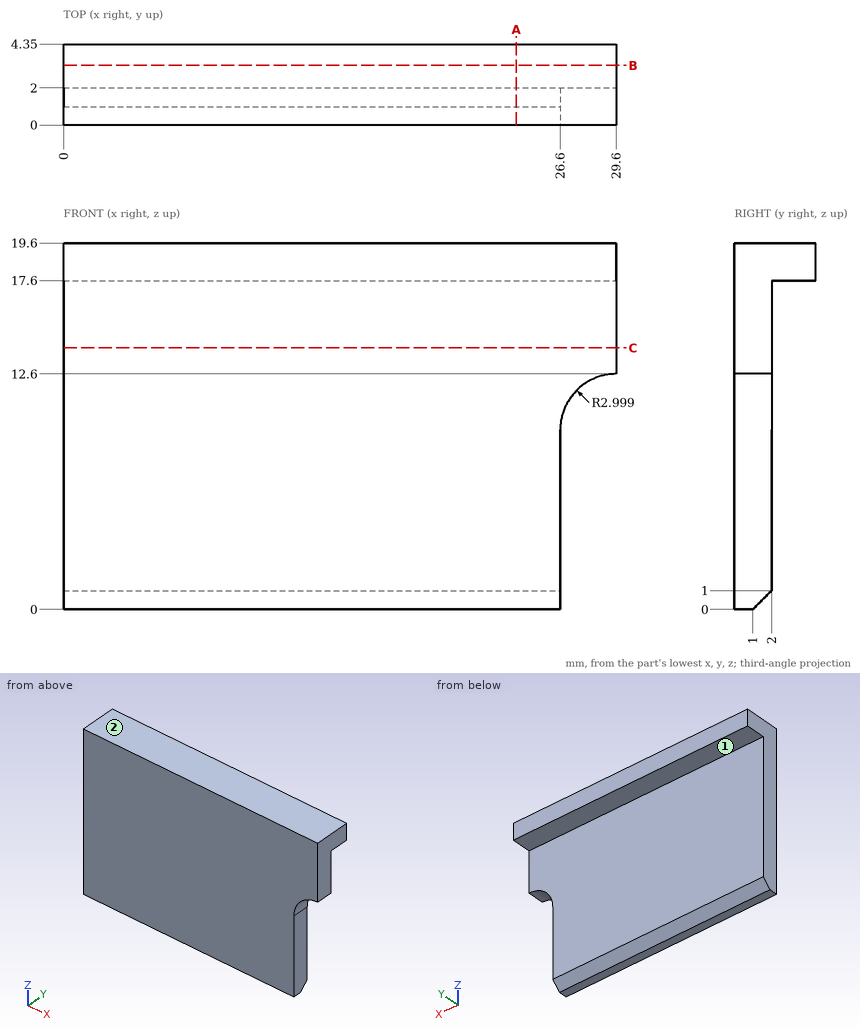
The figure shows three views and two pictorial views of one solid part (mm, origin at its lowest corner). Answer the questions. A direction names the side the tool comes from. Give positions to 0.01 mm unless a question says otherwise; leave off trailing zeros. Loops run counter-clockwise (first coordinate to the right, second up) from the corner with the lowest first, then second, coordinate; pieces in that order, holes last. Notation, with made-up numbers: (-24, 84.5) -> (13, 84.5) arc R14 cw to (13, 104.5) -> close; hole circle Ø3 at (-34, 24). An arc over 180 degrees is marked (long way). Put each result on its own line as item: value. Start each with the question number.
Item 1: The part is cut by section C-C (z = 14). Give the vertices of the cut face in (x, y).
Item 2: Find the intervals of material crossed by L1, parallel to Y at x = 18.5, z = 9.5; L2, parallel to Z at x = 20, y = 2.2; L3, parallel to X at y = 1.1, z = 6.5, in increasing order. Write a range as [from, to].
Item 3: Each of these flat-tipped pins is pushed along its axis until it touches: P1, Ø5, axis at x = 19, z = 6, coming from the +Y side; P2, Ø1.5, axis at x = 22, y = 2.5, coming from the -Z side; P3, Ø1, axis at y = 1, z = 6, coming from the +X side; P4, Ø1, axis at y = 3.5, z = 12, coming from the +X side. Where does it stop, or does it pass through?
Item 4: Which of the six approach directions +Z, -Z, +X, -X, +Y, -Y give full straight-line access (tool end or side, diameter ignored) to the marked faces 1 and 2?
Item 5: The part is cut by section A-A (x = 24.25). Give the vertices of the cut face in (y, z).
Item 6: The part is cut by section B-B (y = 3.2). Give the vertices of the cut face in (x, z).
Answers below:
1. outline: (0, 0) -> (29.6, 0) -> (29.6, 2) -> (0, 2) -> close
2. L1: [0, 2]
2. L2: [17.6, 19.6]
2. L3: [0, 26.6]
3. P1: y = 2
3. P2: z = 0.75
3. P3: x = 26.6
3. P4: through
4. face 1: -Z, +X, -X, +Y
4. face 2: +Z, +X, -X, +Y, -Y
5. outline: (0, 0) -> (1, 0) -> (2, 1) -> (2, 17.6) -> (4.35, 17.6) -> (4.35, 19.6) -> (0, 19.6) -> close
6. outline: (0, 17.6) -> (29.6, 17.6) -> (29.6, 19.6) -> (0, 19.6) -> close
